The listing builds one solid part. Answer for the finished solid, in the listing's coordinates (mm). A direction names the side the tool comes from. Coordinates: 2 decimals unless noted, no trailing zeros. Order: outer loops, then holes, each group sorted by start corner. A loop starts at its lowest first (then second) coordinate and runs counter-clockwise, first axis right, second up. Notation, with made-up numbers: (66, 83) -> (81, 83) arc R27 ccw to (81, 100) -> close; hole circle Ø4 at (89.5, 89.25). An arc over 180 degrees is marked (long way). Write item = value, one per line. Start each with the question number.
```python
from build123d import *

# Parameters (mm, degrees)
F0_R     = 10.5563944733
F4_DEPTH = 17.4
F5_DEPTH = 25


with BuildPart() as f2:
    # F2: sweep along a path in F1
    with BuildLine(Plane.XZ) as f2_path:
        ThreePointArc((32.9693630338, 108.1880107522), (8.9368583588, 86.9712584307), (0, 56.1841763556))
        Line((0, 56.1841763556), (0, 0))
    # F0 (on Top) → F2 (sweep)
    with BuildSketch(Plane.XY):
        Circle(F0_R)
    sweep(path=f2_path.line)

    # F3 (on Front) → F4 (join)
    with BuildSketch(Plane.XZ):
        Polygon((30.7201836258, 128.7439912558), (17.7488774061, 105.8425977826), (60.0541557765, 129.5203427714), (55.4911866784, 139.7707760334), align=None)
    extrude(amount=F4_DEPTH)

    # F3 (on Front) → F5 (join)
    with BuildSketch(Plane.XZ):
        with BuildLine():
            add(Edge.make_bspline(
                [(70.5931460322, 129.5374848512), (72.0787961892, 130.1669103611), (82.3390802937, 134.1470108941), (88.9364784602, 133.4779202279), (87.0999080955, 129.7982594332), (86.9636833649, 129.5641121704)],
                knots=[0.1842071124, 0.1842071124, 0.1842071124, 0.1842071124, 0.1983505917, 0.2859572834, 0.2916534606, 0.2916534606, 0.2916534606, 0.2916534606], degree=3))
            Line((70.5931460322, 129.5374848512), (86.9636833649, 129.5641121704))
        make_face()
        with BuildLine():
            Line((86.9636833649, 129.5641121704), (70.5931460322, 129.5374848512))
            add(Edge.make_bspline(
                [(22.2367271781, 94.8094055057), (21.8099809815, 100.2190570595), (51.2437823198, 121.3397385227), (70.5931460322, 129.5374848512)],
                knots=[0, 0, 0, 0, 0.1842071124, 0.1842071124, 0.1842071124, 0.1842071124], degree=3))
            add(Edge.make_bspline(
                [(55.3720220923, 97.3064601421), (40.8845983612, 95.8756546572), (22.5679207065, 90.6110281103), (22.2367271781, 94.8094055057)],
                knots=[0.8570386708, 0.8570386708, 0.8570386708, 0.8570386708, 1, 1, 1, 1], degree=3))
            add(Edge.make_bspline(
                [(55.3720220923, 97.3064601421), (48.5019136195, 103.4207659246), (49.6477059157, 117.0994626913), (56.8694397807, 119.2096248269)],
                knots=[0.6940672743, 0.6940672743, 0.6940672743, 0.6940672743, 1, 1, 1, 1], degree=3))
            add(Edge.make_bspline(
                [(56.8694397807, 119.2096248269), (65.42174317, 121.7085741266), (82.4951694142, 107.9833870142), (81.0358300805, 100.1313924789)],
                knots=[0, 0, 0, 0, 0.3622993503, 0.3622993503, 0.3622993503, 0.3622993503], degree=3))
            add(Edge.make_bspline(
                [(105.6858077645, 129.5945644379), (107.8117109305, 129.9769098437), (80.0096882515, 114.8143425622), (83.3633906013, 102.5962098802), (81.0358300805, 100.1313924789)],
                knots=[0.512204989, 0.512204989, 0.512204989, 0.512204989, 0.6363641255, 0.7310224434, 0.7310224434, 0.7310224434, 0.7310224434], degree=3))
            add(Edge.make_bspline(
                [(86.9636833649, 129.5641121704), (84.8863296268, 125.9934925799), (65.3812215141, 111.3167629429), (103.3967493158, 129.1828754223), (105.6858077645, 129.5945644379)],
                knots=[0.2916534606, 0.2916534606, 0.2916534606, 0.2916534606, 0.3785170935, 0.512204989, 0.512204989, 0.512204989, 0.512204989], degree=3))
        make_face()
        Polygon((30.7201836258, 128.7439912558), (17.7488774061, 105.8425977826), (60.0541557765, 129.5203427714), (55.4911866784, 139.7707760334), align=None)
        with BuildLine():
            Line((105.6858077645, 129.5945644379), (86.9636833649, 129.5641121704))
            add(Edge.make_bspline(
                [(86.9636833649, 129.5641121704), (84.8863296268, 125.9934925799), (65.3812215141, 111.3167629429), (103.3967493158, 129.1828754223), (105.6858077645, 129.5945644379)],
                knots=[0.2916534606, 0.2916534606, 0.2916534606, 0.2916534606, 0.3785170935, 0.512204989, 0.512204989, 0.512204989, 0.512204989], degree=3))
        make_face()
        with BuildLine():
            add(Edge.make_bspline(
                [(55.3720220923, 97.3064601421), (48.5019136195, 103.4207659246), (49.6477059157, 117.0994626913), (56.8694397807, 119.2096248269)],
                knots=[0.6940672743, 0.6940672743, 0.6940672743, 0.6940672743, 1, 1, 1, 1], degree=3))
            add(Edge.make_bspline(
                [(81.0358300805, 100.1313924789), (77.9372075592, 96.8500433402), (68.1422620706, 98.567673298), (55.3720220923, 97.3064601421)],
                knots=[0.7310224434, 0.7310224434, 0.7310224434, 0.7310224434, 0.8570386708, 0.8570386708, 0.8570386708, 0.8570386708], degree=3))
            add(Edge.make_bspline(
                [(56.8694397807, 119.2096248269), (65.42174317, 121.7085741266), (82.4951694142, 107.9833870142), (81.0358300805, 100.1313924789)],
                knots=[0, 0, 0, 0, 0.3622993503, 0.3622993503, 0.3622993503, 0.3622993503], degree=3))
        make_face()
        with BuildLine():
            add(Edge.make_bspline(
                [(81.0358300805, 100.1313924789), (77.9372075592, 96.8500433402), (68.1422620706, 98.567673298), (55.3720220923, 97.3064601421)],
                knots=[0.7310224434, 0.7310224434, 0.7310224434, 0.7310224434, 0.8570386708, 0.8570386708, 0.8570386708, 0.8570386708], degree=3))
            add(Edge.make_bspline(
                [(81.0358300805, 100.1313924789), (79.6994711252, 92.941095492), (62.8222928035, 90.6758176319), (55.3720220923, 97.3064601421)],
                knots=[0.3622993503, 0.3622993503, 0.3622993503, 0.3622993503, 0.6940672743, 0.6940672743, 0.6940672743, 0.6940672743], degree=3))
        make_face()
    extrude(amount=F5_DEPTH)


solid = f2.part
```
Item 1: For a pull along X with two mould halves and no side action, classify faces 1 (the flat face through (24.325, -12.325, 117.454)), 2 (the flat face through (33.032, 2.198, 108.054)), 3 (the flat face through (57.805, -12.325, 134.574)), 4 (the cylindrical face through (-7.781, -7.135, 27.699)) as pulls with the +X half, pulls with the -X half, needs draft (parallel to the pull), parting line crosses it, or undercut.
Item 2: Each of these flat-tipped pins is pushed along its axis until it touches: pin 1 (10 mm diameter, centred on x = 27, y = 7, fed in from -Z); pin 2 (20 mm diameter, centred on x = 84, z = 122.5, fed in from +Y); pin 3 (4 mm diameter, centred on x = 87, y = 1, fed in from +Z); pin 4 (1 mm diameter, centred on y = -12.5, z = 15.5, fed in from +X). Where does it stop, or does it pass through?
Item 3: Which of the six approach directions +Z, -Z, +X, -X, +Y, -Y give full straight-line access (tool end or side, diameter ignored) to faces 5 (the flat face through (38.61, -12.32, 117.52)), 6 (the flat face through (0, 0, 0))?
Item 4: Consider probe 1 along X at (y, z) = (-17, 126); probe 2 along Z at (x, y) = (38, -18); probe 3 along Z at (x, y) = (50, -12). Determine where each line is inside the solid, lowest interval first.
Item 5: Section A-A, the plane z = 38 is taken. Give the vertices of the cut face in (x, y), then the cut area to 3 significant figures.
A:
q1.face_1 = pulls with the -X half
q1.face_2 = undercut
q1.face_3 = undercut
q1.face_4 = parting line crosses it
q2.pin_1 = 89.13
q2.pin_2 = 0
q2.pin_3 = 132.95
q2.pin_4 = through
q3.face_5 = -Y
q3.face_6 = -Z, +X, -X, +Y, -Y
q4.probe_1 = 29.17 to 53.76, 63.11 to 100.88
q4.probe_2 = 94.68 to 110.41, 117.18 to 131.98
q4.probe_3 = 96.64 to 118.49, 123.89 to 137.33
q5.outline = circle Ø21.11 at (0, 0)
q5.area = 350 mm^2
